```python
from build123d import *

# Parameters (mm, degrees)
SKETCH007_W   = 44.6
SKETCH007_H   = 24.4
SKETCH007_W_2 = 40.6
SKETCH007_H_2 = 20.4
PAD006_DEPTH  = 18
BOX001_W      = 44.6
BOX001_H      = 24.2
BOX001_DEPTH  = 2
BOX002_W      = 40.6
BOX002_H      = 3
BOX002_DEPTH  = 8


with BuildPart() as part:
    # Sketch007 → Pad006 (new body)
    with BuildSketch(Plane.XY):
        with Locations((20.3, 10.2)):
            Rectangle(SKETCH007_W, SKETCH007_H)
        with Locations((20.3, 10.2)):
            Rectangle(SKETCH007_W_2, SKETCH007_H_2, mode=Mode.SUBTRACT)
    extrude(amount=-PAD006_DEPTH)

    # Box001 → Box001 (join)
    with BuildSketch(Plane(origin=(-2, -2, -2), x_dir=(1, 0, 0), z_dir=(0, 0, 1))):
        with Locations((22.3, 12.1)):
            Rectangle(BOX001_W, BOX001_H)
    extrude(amount=BOX001_DEPTH)

    # Box002 → Box002 (cut)
    with BuildSketch(Plane(origin=(0, 20, -18), x_dir=(1, 0, 0), z_dir=(0, 0, 1))):
        with Locations((20.3, 1.5)):
            Rectangle(BOX002_W, BOX002_H)
    extrude(amount=BOX002_DEPTH, mode=Mode.SUBTRACT)


solid = part.part
```
Source: CAD feature listing. Evaluate the final solid. Frame: model axes, mm. A direction names the side the tool comes from. Coordinates: 2 decimals unless noted, no trailing zeros. Loops run counter-clockwise (first coordinate to the right, second up) from the corner with the lowest first, then second, coordinate; pieces in that order, holes last. Notation, with made-up numbers: M 74,82 L 81,82 A23 ccw 81,94 Z; hole C -15.75,24 d6. An arc over 180 degrees is marked long. Put each result on its own line as item: value. Start each with the question number.
1) Cut plane A-A on z = -4. Return the cut outline in (x, y), then the cut area to 3 significant figures.
2) Ray query, L1, parallel to X at y = 3, z = -6.25; L2, parallel to Y at x = 1.5, z = -7.5; L3, parallel to Z at x = 20, y = 0.75. Return the intervals inside material, ascending. Write a range as from..to.
3) Reachability of faces 1 (the face through (20, 21, -10)), 2 (the face through (20, -1, -18)), 3 (the face through (20, 0, -10)) from +Z, -Z, +X, -X, +Y, -Y: full face, straight path, thin tool, end or side. Return the list, or none.
4) Cut plane B-B on x = 18. Return the cut outline in (y, z), then the cut area to 3 significant figures.
5) Contact query for flat-ended pins moving along their axis: pin 1 Ø10 at (x, y) = (19, 13.5) entering from -Z; pin 2 Ø1 at (x, y) = (14, 21) entering from -Z. Output: stop coordinate, or through.
6) Cut plane C-C on y = 6. Return the cut outline in (x, z), then the cut area to 3 significant figures.
7) Pull-direction query (X, two-part tool) for faces 4 (the face through (-2, 10, -9)), 5 (the face through (20, 20.4, -6)), 6 (the face through (20, 10, 0)), 7 (the face through (42.6, 10, -9)); classes: pulls with the +X half, pulls with the -X half, needs draft (parallel to the pull), parting line crosses it, or undercut.
The answers:
1. outline: M -2,-2 L 42.6,-2 L 42.6,22.4 L -2,22.4 Z; hole M 0,0 L 40.6,0 L 40.6,20.4 L 0,20.4 Z
1. area: 260 mm²
2. L1: x = -2..0, 40.6..42.6
2. L2: y = -2..0, 20.4..22.4
2. L3: z = -2..0
3. face 1: -Z, +Y
3. face 2: -Z, +X, -X, +Y, -Y
3. face 3: -Z
4. outline: M -2,-18 L 0,-18 L 0,-2 L 20.4,-2 L 20.4,-10 L 22.4,-10 L 22.4,0 L -2,0 Z
4. area: 96.8 mm²
5. pin 1: stops at z = -2
5. pin 2: stops at z = -10
6. outline: M -2,-18 L 0,-18 L 0,-2 L 40.6,-2 L 40.6,-18 L 42.6,-18 L 42.6,0 L -2,0 Z
6. area: 153 mm²
7. face 4: pulls with the -X half
7. face 5: undercut
7. face 6: needs draft
7. face 7: pulls with the +X half
